from build123d import *

# Parameters (mm, degrees)
SKETCH_1_R          = 1.6
EXTRUDE_4_DEPTH     = 3
SKETCH_2_W          = 40
SKETCH_2_H          = 3
EXTRUDE_5_DEPTH     = 43
SKETCH_3_R          = 1.6
CUT_EXTRUDE_1_DEPTH = 63.306805946
FILLET_5_R          = 2
FILLET_6_R          = 2
FILLET_7_R          = 2


with BuildPart() as part:
    # 草图1 → 凸台-拉伸4 (new body)
    with BuildSketch(Plane.XY):
        with BuildLine():
            Line((-17.213055582, 18.908780902), (-17.213055582, -5.203950579))
            Line((-17.213055582, -5.203950579), (22.786944418, -5.203950579))
            Line((22.786944418, -5.203950579), (22.786944418, 18.908780902))
            ThreePointArc((22.786944418, 18.908780902), (2.786944418, 38.908780902), (-17.213055582, 18.908780902))
        make_face()
        with Locations((-4.94763916, 5.557362749)):
            Circle(SKETCH_1_R, mode=Mode.SUBTRACT)
        with Locations((10.539247833, 5.319833808)):
            Circle(SKETCH_1_R, mode=Mode.SUBTRACT)
        with Locations((-12.656689842, 18.908780902)):
            Circle(SKETCH_1_R, mode=Mode.SUBTRACT)
        with Locations((-5.045757748, 32.297473855)):
            Circle(SKETCH_1_R, mode=Mode.SUBTRACT)
        with BuildLine():
            ThreePointArc((9.343310158, 10.296049421), (2.843310158, 3.796049421), (-3.656689842, 10.296049421))
            Line((-3.656689842, 10.296049421), (-3.656689842, 24.296049421))
            ThreePointArc((-3.656689842, 24.296049421), (2.843310158, 30.796049421), (9.343310158, 24.296049421))
            Line((9.343310158, 24.296049421), (9.343310158, 10.296049421))
        make_face(mode=Mode.SUBTRACT)
        with Locations((18.343310158, 18.908780902)):
            Circle(SKETCH_1_R, mode=Mode.SUBTRACT)
        with Locations((10.586753622, 32.160604209)):
            Circle(SKETCH_1_R, mode=Mode.SUBTRACT)
    extrude(amount=EXTRUDE_4_DEPTH)

    # 草图2 → 凸台-拉伸5 (add)
    with BuildSketch(Plane.XY):
        with Locations((2.786944418, -6.703950579)):
            Rectangle(SKETCH_2_W, SKETCH_2_H)
    extrude(amount=EXTRUDE_5_DEPTH)

    # 草图3 → 切除-拉伸1 (cut, through all)
    with BuildSketch(Plane(origin=(0, 0, 0), x_dir=(1, 0, 0), z_dir=(0, 1, 0))):
        with Locations(Location((-12.213055582, -35, 0), (0, 0, 270))):
            Circle(SKETCH_3_R)
        with Locations(Location((17.786944418, -35, 0), (0, 0, 270))):
            Circle(SKETCH_3_R)
        with Locations(Location((17.786944418, -11, 0), (0, 0, 270))):
            Circle(SKETCH_3_R)
        with Locations(Location((-12.213055582, -11, 0), (0, 0, 270))):
            Circle(SKETCH_3_R)
    extrude(amount=-CUT_EXTRUDE_1_DEPTH, mode=Mode.SUBTRACT)

    # 圆角5
    fillet_5_edges = [part.edges().sort_by_distance(p)[0] for p in [
        (22.786944418, -6.703950579, 43),
    ]]
    fillet(fillet_5_edges, radius=FILLET_5_R)

    # 圆角6
    fillet_6_edges = [part.edges().sort_by_distance(p)[0] for p in [
        (-17.213055582, -6.703950579, 43),
    ]]
    fillet(fillet_6_edges, radius=FILLET_6_R)

    # 圆角7
    fillet_7_edges = [part.edges().sort_by_distance(p)[0] for p in [
        (2.786944418, -8.203950579, 0),
    ]]
    fillet(fillet_7_edges, radius=FILLET_7_R)


solid = part.part
Can you work these out from the model? Positions are in its coordinate system, mm. A direction names the side the tool comes from. Give positions to 0.01 mm unless a question says otherwise; leave off trailing zeros. Loops run counter-clockwise (first coordinate to the right, second up) from the corner with the lowest first, then second, coordinate; pieces in that order, holes last. Notation, with made-up numbers: M 19,46.5 L 53,46.5 A10 ccw 53,52.5 Z; hole C 76.25,-19 d1. An arc over 180 degrees is marked long. One line per item, written item: value. Start each with the question number.
1) If we section it at C-C, the plane x = 6: Write out the boundary of the cut face in (y, z).
2) If we section it at B-B, the plane y = 8: Write out the boundary of the cut face in (x, z).
3) On a 3-axis mill with a long thin cutter (end or side, diameter ignored), from which of +Z, -Z, +X, -X, +Y, -Y can I reach the whole of each face in a straight line? I mean faces 4 (the face through (-11.13, -6.68, 33.82)), 5 (the face through (9.343, 17, 1)), 6 (the face through (11, 12, 3)). Say none if no direction works.
4) If I drill on line 1 (X direction, y = -7.55, z = 35); line 2 (Y direction, x = 6.5, z = 24); line 3 (Z direction, x = 10, y = 13), over which ranges is the centre line in solid material (lowest first)? Write a range as [from, to].
5) I'm going to push flat-ended pins straight in: pin 1 (3.5 mm diameter, centred on x = -5.05, y = 32.3, fed in from -Z); pin 2 (2 mm diameter, centred on x = -3.5, y = -1.5, fed in from +Z); pin 3 (3 mm diameter, centred on x = -12.66, y = 18.91, fed in from +Z). Where does each tip first touch, or does it pass through?
6) If we section it at A-A, the plane z = 11: Write out the boundary of the cut face in (x, y).
7) Thinking about a two-plate mould opening in Y: for faces 1 (the face through (-16.61, -6.68, 42.43)), 2 (the face through (3, -8.204, 22)), 3 (the face through (-4.09, 6.91, 1.48)), which applies, +Y half, -Y half, draft (parallel to the pull), parting line (faces both ways), or undercut?
8) If we section it at D-D, the plane y = 3: Write out the boundary of the cut face in (x, z), and give its area (3 significant figures).
Completed:
1. outline: M -8.2,2 A2 ccw -6.2,0 L 4.61,0 L 4.61,3 L -5.2,3 L -5.2,43 L -8.2,43 Z; M 29.98,0 L 38.65,0 L 38.65,3 L 29.98,3 Z
2. outline: M -17.21,0 L -3.24,0 L -3.24,3 L -17.21,3 Z; M 8.92,0 L 22.79,0 L 22.79,3 L 8.92,3 Z
3. face 4: +Y, -Y
3. face 5: +Z, -Z
3. face 6: +Z, +X, -X, +Y
4. line 1: x = [-17.21, -13.81], [-10.61, 16.19], [19.39, 22.79]
4. line 2: y = [-8.2, -5.2]
4. line 3: z = [0, 3]
5. pin 1: stops at z = 0
5. pin 2: stops at z = 3
5. pin 3: passes through
6. outline: M -17.21,-8.2 L -13.81,-8.2 L -13.81,-5.2 L -17.21,-5.2 Z; M -10.61,-8.2 L 16.19,-8.2 L 16.19,-5.2 L -10.61,-5.2 Z; M 19.39,-8.2 L 22.79,-8.2 L 22.79,-5.2 L 19.39,-5.2 Z
7. face 1: draft
7. face 2: -Y half
7. face 3: undercut
8. outline: M -17.21,0 L 22.79,0 L 22.79,3 L -17.21,3 Z
8. area: 120 mm^2
